```python
from build123d import *

# Parameters (mm, degrees)
BASE_BODY_DEPTH         = 5
BASE_BODY_DEPTH_BACK    = 7.2
BASE_BODY_SKETCH_R      = 4.8
RBODY_SML_SKETCH_R      = 3.3
RBODY_SML_DEPTH         = 5.5
HEX_2_DEPTH             = 3
THREAD_OFFSET_START     = -7.5
THREAD_OFFSET_SKETCH_R  = 3.5
THREAD_OFFSET_DEPTH     = 0.3
THREAD_SKETCH_W         = 2.5
THREAD_SKETCH_H         = 5.1
CHAMFER_2_SIZE          = 0.25
RBODY_SKETCH_R          = 4.65
RBODY_DEPTH             = 9.7
TUBE_SKETCH_R           = 2
TUBE_DEPTH              = 12.7
TUBE_RADIUS_R           = 0.5
DIAMETER_R              = 1
BODY_CHAMFER_SIZE       = 0.25
TAMPER_BODY_SKETCH_R    = 3.9166745
TAMPER_BODY_DEPTH       = 10.7
TAMPER_BODY_CHAM_SIZE   = 0.375
TAMPER_CONTROL_SKETCH_R = 2.725
TAMPER_CONTROL_DEPTH    = 0.75
TAMPER_FLAT_DEPTH       = 1.5


with BuildPart() as part:
    # Base-Body_Sketch → Base-Body (new, two sides: drawn at the far end of the back side and taken through both)
    with BuildSketch(Plane(origin=(0, 0, 0), x_dir=(1, 0, 0), z_dir=(0, 1, 0)).offset(-BASE_BODY_DEPTH_BACK)):
        with Locations(Location((0, 0, 0), (0, 0, 270))):
            Circle(BASE_BODY_SKETCH_R)
    extrude(amount=BASE_BODY_DEPTH + BASE_BODY_DEPTH_BACK)

    # RBody_sml_Sketch → RBody_sml (add)
    with BuildSketch(Plane(origin=(0, 0, 0), x_dir=(0, 0, -1), z_dir=(1, 0, 0))):
        Circle(RBODY_SML_SKETCH_R)
    extrude(amount=-RBODY_SML_DEPTH)

    # Hex_Sketch → Hex 2 (add)
    with BuildSketch(Plane(origin=(0, 5, 0), x_dir=(-1, 0, 0), z_dir=(0, 1, 0))):
        Polygon((4, 2.309401077), (0, 4.618802154), (-4, 2.309401077), (-4, -2.309401077), (0, -4.618802154), (4, -2.309401077), align=None)
    extrude(amount=HEX_2_DEPTH)

    # Hex_Chamfer_Sketch → Hex_Chamfer (revolve, cut)
    with BuildSketch(Plane(origin=(0, 0, 0), x_dir=(0, 0, -1), z_dir=(1, 0, 0))):
        Polygon((4, 8), (4.618802154, 8), (4.618802154, 7.64273441), align=None)
    revolve(axis=Axis((0, 0, 0), (0, 1, 0)), mode=Mode.SUBTRACT)

    # Thread_Offset_Sketch (on Top Plane) → Thread_Offset (add)
    with BuildSketch(Plane(origin=(0, 0, 0), x_dir=(1, 0, 0), z_dir=(0, 1, 0)).offset(THREAD_OFFSET_START)):
        with Locations(Location((0, 0, 0), (0, 0, 270))):
            Circle(THREAD_OFFSET_SKETCH_R)
    extrude(amount=THREAD_OFFSET_DEPTH)

    # Thread_Sketch → Thread (revolve)
    with BuildSketch(Plane.XY, mode=Mode.PRIVATE) as thread_sk:
        with Locations((-1.25, -9.75)):
            Rectangle(THREAD_SKETCH_W, THREAD_SKETCH_H)
    revolve(thread_sk.sketch.rotate(Axis((0, 0, 0), (0, -1, 0)), 270), axis=Axis((0, 0, 0), (0, -1, 0)))

    # Chamfer 2: size read off the stored shape
    # Chamfer 2
    chamfer_2_edges = [part.edges().sort_by_distance(p)[0] for p in [
        (0, -12.3, -2.5),
    ]]
    chamfer(chamfer_2_edges, length=CHAMFER_2_SIZE)

    # RBody_Sketch → RBody (add)
    with BuildSketch(Plane(origin=(-5.5, 0, 0), x_dir=(0, 0, -1), z_dir=(1, 0, 0))):
        Circle(RBODY_SKETCH_R)
    extrude(amount=-RBODY_DEPTH)

    # Release_Sketch → Release (revolve)
    with BuildSketch(Plane.XY, mode=Mode.PRIVATE) as release_sk:
        with BuildLine():
            Line((-17.3, 0), (-17.3, 4.05))
            ThreePointArc((-17.3, 4.05), (-17.153553391, 4.403553391), (-16.8, 4.55))
            Line((-16.8, 4.55), (-15.8, 4.55))
            Line((-15.8, 4.55), (-15.8, 2.5))
            Line((-15.8, 2.5), (-15.2, 2.5))
            Line((-15.2, 2.5), (-15.2, 0))
            Line((-15.2, 0), (-17.3, 0))
        make_face()
    revolve(release_sk.sketch.rotate(Axis((0, 0, 0), (-1, 0, 0)), 90), axis=Axis((0, 0, 0), (-1, 0, 0)))

    # Tube_Sketch → Tube (cut)
    with BuildSketch(Plane(origin=(-17.3, 0, 0), x_dir=(0, 0, -1), z_dir=(1, 0, 0))):
        Circle(TUBE_SKETCH_R)
    extrude(amount=TUBE_DEPTH, mode=Mode.SUBTRACT)

    # Tube_Radius
    tube_radius_edges = [part.edges().sort_by_distance(p)[0] for p in [
        (-17.3, 0, 2),
    ]]
    fillet(tube_radius_edges, radius=TUBE_RADIUS_R)

    # RBody_Chamfer: read off the stored shape, not the designer's step
    # RBody_Chamfer outline → RBody_Chamfer (revolve, cut)
    with BuildSketch(Plane.YX):
        Polygon((4.65, -5.5), (3.3, -5.5), (4.65, -5.991359816), align=None)
    revolve(axis=Axis((0, 0, 0), (1, 0, 0)), mode=Mode.SUBTRACT)

    # Port: sweep along a path in Profile
    with BuildLine(Plane.XY) as port_path:
        Line((-17.3, 0), (-2, 0))
        ThreePointArc((-2, 0), (-0.585786438, -0.585786438), (0, -2))
        Line((0, -2), (0, -12.3))
    # Diameter → Port (sweep, cut)
    with BuildSketch(Plane(origin=(0, -12.3, 0), x_dir=(-1, 0, 0), z_dir=(0, 1, 0))):
        Circle(DIAMETER_R)
    sweep(path=port_path.line, mode=Mode.SUBTRACT)

    # Body_Chamfer
    # the kernel refuses this chamfer: 0.25 mm, written as the material it takes off along each edge
    with BuildSketch(Plane(origin=(0, -7.2, 0), x_dir=(0, 0, 1), z_dir=(-1, 0, 0))) as body_chamfer_piece_1:
        Polygon((4.8, BODY_CHAMFER_SIZE), (4.8 - BODY_CHAMFER_SIZE, 0), (4.8, 0), align=None)
    revolve(axis=Axis((0, -7.2, 0), (0, 1, 0)), mode=Mode.SUBTRACT)
    with BuildSketch(Plane(origin=(0, 5, 0), x_dir=(0, 0, 1), z_dir=(-1, 0, 0))) as body_chamfer_piece_2_section:
        Polygon((4.8, -BODY_CHAMFER_SIZE), (4.8 - BODY_CHAMFER_SIZE, 0), (4.8, 0), align=None)
    body_chamfer_piece_2 = revolve(axis=Axis((0, 5, 0), (0, 1, 0)), mode=Mode.PRIVATE)
    body_chamfer_piece_2 = split(body_chamfer_piece_2, bisect_by=Plane(origin=(2, 5, 3.464101615), z_dir=(0.5000000000000002, 0, 0.8660254037844385)), keep=Keep.TOP, mode=Mode.PRIVATE)
    add(body_chamfer_piece_2, mode=Mode.SUBTRACT)
    with BuildSketch(Plane(origin=(0, 5, 0), x_dir=(0, 0, 1), z_dir=(-1, 0, 0))) as body_chamfer_piece_3_section:
        Polygon((4.8, -BODY_CHAMFER_SIZE), (4.8 - BODY_CHAMFER_SIZE, 0), (4.8, 0), align=None)
    body_chamfer_piece_3 = revolve(axis=Axis((0, 5, 0), (0, 1, 0)), mode=Mode.PRIVATE)
    body_chamfer_piece_3 = split(body_chamfer_piece_3, bisect_by=Plane(origin=(-2, 5, 3.464101615), z_dir=(-0.49999999999999983, 0, 0.8660254037844388)), keep=Keep.TOP, mode=Mode.PRIVATE)
    add(body_chamfer_piece_3, mode=Mode.SUBTRACT)
    with BuildSketch(Plane(origin=(0, 5, 0), x_dir=(0, 0, 1), z_dir=(-1, 0, 0))) as body_chamfer_piece_4_section:
        Polygon((4.8, -BODY_CHAMFER_SIZE), (4.8 - BODY_CHAMFER_SIZE, 0), (4.8, 0), align=None)
    body_chamfer_piece_4 = revolve(axis=Axis((0, 5, 0), (0, 1, 0)), mode=Mode.PRIVATE)
    body_chamfer_piece_4 = split(body_chamfer_piece_4, bisect_by=Plane(origin=(4, 5, 0), z_dir=(1, 0, 0)), keep=Keep.TOP, mode=Mode.PRIVATE)
    add(body_chamfer_piece_4, mode=Mode.SUBTRACT)
    with BuildSketch(Plane(origin=(0, 5, 0), x_dir=(0, 0, 1), z_dir=(-1, 0, 0))) as body_chamfer_piece_5_section:
        Polygon((4.8, -BODY_CHAMFER_SIZE), (4.8 - BODY_CHAMFER_SIZE, 0), (4.8, 0), align=None)
    body_chamfer_piece_5 = revolve(axis=Axis((0, 5, 0), (0, 1, 0)), mode=Mode.PRIVATE)
    body_chamfer_piece_5 = split(body_chamfer_piece_5, bisect_by=Plane(origin=(-4, 5, 0), z_dir=(-1, 0, 0)), keep=Keep.TOP, mode=Mode.PRIVATE)
    add(body_chamfer_piece_5, mode=Mode.SUBTRACT)
    with BuildSketch(Plane(origin=(0, 5, 0), x_dir=(0, 0, 1), z_dir=(-1, 0, 0))) as body_chamfer_piece_6_section:
        Polygon((4.8, -BODY_CHAMFER_SIZE), (4.8 - BODY_CHAMFER_SIZE, 0), (4.8, 0), align=None)
    body_chamfer_piece_6 = revolve(axis=Axis((0, 5, 0), (0, 1, 0)), mode=Mode.PRIVATE)
    body_chamfer_piece_6 = split(body_chamfer_piece_6, bisect_by=Plane(origin=(2, 5, -3.464101615), z_dir=(0.4999999999999999, 0, -0.8660254037844388)), keep=Keep.TOP, mode=Mode.PRIVATE)
    add(body_chamfer_piece_6, mode=Mode.SUBTRACT)
    with BuildSketch(Plane(origin=(0, 5, 0), x_dir=(0, 0, 1), z_dir=(-1, 0, 0))) as body_chamfer_piece_7_section:
        Polygon((4.8, -BODY_CHAMFER_SIZE), (4.8 - BODY_CHAMFER_SIZE, 0), (4.8, 0), align=None)
    body_chamfer_piece_7 = revolve(axis=Axis((0, 5, 0), (0, 1, 0)), mode=Mode.PRIVATE)
    body_chamfer_piece_7 = split(body_chamfer_piece_7, bisect_by=Plane(origin=(-2, 5, -3.464101615), z_dir=(-0.5, 0, -0.8660254037844387)), keep=Keep.TOP, mode=Mode.PRIVATE)
    add(body_chamfer_piece_7, mode=Mode.SUBTRACT)

    # Tamper Body_Sketch → Tamper Body (add)
    with BuildSketch(Plane(origin=(0, 8, 0), x_dir=(-1, 0, 0), z_dir=(0, 1, 0))):
        with Locations(Location((0, 0, 0), (0, 0, 270))):
            Circle(TAMPER_BODY_SKETCH_R)
    extrude(amount=TAMPER_BODY_DEPTH)

    # Tamper Body Cham
    tamper_body_cham_edges = [part.edges().sort_by_distance(p)[0] for p in [
        (0, 18.7, 3.9166745),
    ]]
    chamfer(tamper_body_cham_edges, length=TAMPER_BODY_CHAM_SIZE)

    # Tamper Control_Sketch → Tamper Control (cut)
    with BuildSketch(Plane(origin=(0, 18.7, 0), x_dir=(-1, 0, 0), z_dir=(0, 1, 0))):
        with Locations(Location((0, 0, 0), (0, 0, 90))):
            Circle(TAMPER_CONTROL_SKETCH_R)
    extrude(amount=-TAMPER_CONTROL_DEPTH, mode=Mode.SUBTRACT)

    # Tamper Flat_Sketch → Tamper Flat (cut)
    with BuildSketch(Plane(origin=(0, 17.95, 0), x_dir=(-1, 0, 0), z_dir=(0, 1, 0))):
        with BuildLine():
            Line((0.35, -2.323790008), (0.35, 2.323790008))
            ThreePointArc((0.35, 2.323790008), (0, 2.35), (-0.35, 2.323790008))
            Line((-0.35, 2.323790008), (-0.35, -2.323790008))
            ThreePointArc((-0.35, -2.323790008), (0, -2.35), (0.35, -2.323790008))
        make_face()
    extrude(amount=-TAMPER_FLAT_DEPTH, mode=Mode.SUBTRACT)


solid = part.part
```
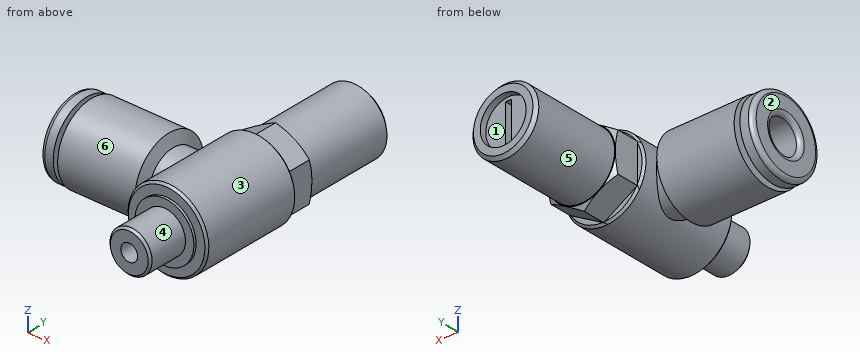
For this review, take the finished solid that the model builds, in its own axes (mm). Face numbers are marked on the shaded views. A direction names the side the tool comes from. Coordinates: 2 decimals unless noted, no trailing zeros. Loops run counter-clockwise (first coordinate to the right, second up) from the corner with the lowest first, then second, coordinate; pieces in that order, holes last.
1. For line 1 (X direction, y = 3, z = -3); line 2 (X direction, y = 18.25, z = 0) (3 decimals); line 3 (Z direction, x = 0, y = -6), list the stretches that pass through material, from the lowest coordinate up.
2. Insertion check: P1, Ø12, axis at x = -14.5, y = -7, coming from the +Z side; P2, Ø5, axis at y = 1, z = -1.5, coming from the -X side; P3, Ø5, axis at y = 3.5, z = -3.5, coming from the +X side; P4, Ø4, axis at x = -11.5, z = 3, coming from the -Y side. Each pin has a flat end and moves straight along its axis. Give the tip position at first contact, or say it passes through.
3. Add section A-A, the plane x = -14.5. Give the boundary of the cut face in (y, z).
4. Add section B-B, the plane y = 15.5. Give the boundary of the cut face in (x, z).
5. For the marked faces 4, 5 and 6, list the 3-axis set-ups (+Z, -Z, +X, -X, +Y, -Y) from which the entire face can be reached by the end or side of a thin tool; tool diameter is ignored.
6. Mouldability with a two-part tool opening along Z and no side actions: class the marked faces 1, 2 and 3 as +Z half, -Z half, draft (parallel to the pull), parting line (faces both ways), or undercut.
Result:
1. line 1: x = -17.26 to -15.8, -15.2 to -5.84, -3.75 to 3.75
1. line 2: x = -3.917 to -2.725, 2.725 to 3.917
1. line 3: z = -4.8 to -1, 1 to 4.8
2. P1: stops at z = 4.54
2. P2: stops at x = -17.3
2. P3: stops at x = 4.69
2. P4: stops at y = -4.54
3. outline: circle Ø9.3 at (0, 0); hole circle Ø4 at (0, 0)
4. outline: circle Ø7.83 at (0, 0)
5. face 4: -Y
5. face 5: +Y
5. face 6: -X
6. face 1: undercut
6. face 2: draft
6. face 3: parting line
